Source: CAD feature listing. Evaluate the final solid. Frame: model axes, mm. A direction names the side the tool comes from. Coordinates: 2 decimals unless noted, no trailing zeros. Order: outer loops, then holes, each group sorted by start corner. A loop starts at its lowest first (then second) coordinate and runs counter-clockwise, first axis right, second up. Notation, with made-up numbers: (57.25, 80.25) -> (69.25, 80.25) arc R15 ccw to (69.25, 87.25) -> close; hole circle Ø6 at (74.25, 59.25). An arc over 180 degrees is marked (long way). Write item = value, one per line. Start each with the question number.
Item 1: Section query A-A (x = 0). Output: boundary loops of the cut face in (y, z).
Item 2: Section query B-B (y = -4.5). Output: boundary loops of the cut face in (x, z), then the cut area to 3 significant figures.
Item 3: Ray query, line 1 along Y through (x, z) = (-1.7, -1.5); line 2 along Y through (x, z) = (0.95, 0.65); line 3 along X through (y, z) = (-5.25, 0). Return the intervals inside material, ascending. Write a range as [from, to].
Item 4: Contact query for flat-ended pins moving along their axis: pin 1 (2 mm diameter, centred on x = -1, y = 4.5, fed in from -Z); pin 2 (2 mm diameter, centred on x = 2, y = 3, fed in from -Z). Output: stop coordinate, or through.
Item 5: Set-up query: faces 5 (the flat face through (0, 8, -1.5)), 6 (the flat face through (2, 6, 0)), 7 (the cylindrical face through (-0.54, 7.52, 2.44)). Return all of +Z, -Z, +X, -X, +Y, -Y with unobstructed straight access to the full face (end or side cutting, diameter ignored); none if empty.
Item 6: Mould query, pull axis X, two halves, no side actions, for faces 1 (the flat face through (0, 9, -2)), 2 (the cylindrical face through (-1.5, -1.39, -0.07)), 3 (the flat face through (-1.293, 8.014, -0.76)), 4 (the flat face through (-1.305, 8.014, 0.74)). Classes: released by +X, released by -X, zero draft, split by the parting line, or undercut.
```python
from build123d import *

# Parameters (mm, degrees)
CUT_EXTRUDE1_DEPTH = 2
FILLET1_R          = 0.25


with BuildPart() as part:
    # Sketch1 → Revolve1 (revolve)
    with BuildSketch(Plane.XY):
        Polygon((0, -9), (1.5, -9), (1.5, 6), (2.5, 6), (2.5, 9), (0, 9), align=None)
    revolve(axis=Axis((0, -1000, 0), (0, 1, 0)))

    # Sketch2 → Cut-Extrude1 (cut)
    with BuildSketch(Plane(origin=(0, 9, 0), x_dir=(1, 0, 0), z_dir=(0, 1, 0))):
        Polygon((0.866025404, 1.5), (-0.866025404, 1.5), (-1.732050808, 0), (-0.866025404, -1.5), (0.866025404, -1.5), (1.732050808, 0), align=None)
    extrude(amount=-CUT_EXTRUDE1_DEPTH, mode=Mode.SUBTRACT)

    # Fillet1
    fillet1_edges = [part.edges().sort_by_distance(p)[0] for p in [
        (-2.5, 9, 0),
        (-2.5, 6, 0),
    ]]
    fillet(fillet1_edges, radius=FILLET1_R)


solid = part.part
```
Computed:
q1.outline = (-9, -1.5) -> (6, -1.5) -> (6, -2.25) arc R0.25 ccw to (6.25, -2.5) -> (8.75, -2.5) arc R0.25 ccw to (9, -2.25) -> (9, -1.5) -> (7, -1.5) -> (7, 1.5) -> (9, 1.5) -> (9, 2.25) arc R0.25 ccw to (8.75, 2.5) -> (6.25, 2.5) arc R0.25 ccw to (6, 2.25) -> (6, 1.5) -> (-9, 1.5) -> close
q2.outline = circle Ø3 at (0, 0)
q2.area = 7.07 mm^2
q3.line_1 = [6, 9]
q3.line_2 = [-9, 7]
q3.line_3 = [-1.5, 1.5]
q4.pin_1 = -1.5
q4.pin_2 = -1.12
q5.face_5 = +Y
q5.face_6 = -Y
q5.face_7 = +Y, -Y
q6.face_1 = zero draft
q6.face_2 = split by the parting line
q6.face_3 = undercut
q6.face_4 = undercut
